from build123d import *

# Parameters (mm, degrees)
CUT_EXTRUDE2_DEPTH      = 87.677563418
CUT_EXTRUDE2_DEPTH_BACK = 87.677563418
SKETCH3_W               = 4
SKETCH3_H               = 2.8


with BuildPart() as part:
    # Sketch1 → Revolve1 (revolve)
    with BuildSketch(Plane.XY, mode=Mode.PRIVATE) as revolve1_sk:
        with BuildLine():
            Line((0, 0), (55, 0))
            Line((55, 0), (55, 8.5))
            Line((55, 8.5), (1, 8.5))
            ThreePointArc((1, 8.5), (0.292893219, 8.792893219), (0, 9.5))
            Line((0, 9.5), (0, 12))
            Line((0, 12), (-30, 12))
            Line((-30, 12), (-30, 9.5))
            ThreePointArc((-30, 9.5), (-30.292893219, 8.792893219), (-31, 8.5))
            Line((-31, 8.5), (-85, 8.5))
            Line((-85, 8.5), (-85, 0))
            Line((-85, 0), (0, 0))
        make_face()
    revolve(revolve1_sk.sketch.rotate(Axis((-85, 0, 0), (1, 0, 0)), 180), axis=Axis((-85, 0, 0), (1, 0, 0)))

    # Sketch3 → Cut-Extrude2 (cut, two sides: drawn at the far end of the back side and taken through both)
    with BuildSketch(Plane(origin=(0, 0, 0), x_dir=(0, 0, -1), z_dir=(1, 0, 0)).offset(-CUT_EXTRUDE2_DEPTH_BACK)):
        with Locations((2, 9.913708499)):
            Rectangle(SKETCH3_W, SKETCH3_H)
        with Locations((-2, 9.913708499)):
            Rectangle(SKETCH3_W, SKETCH3_H)
        with BuildLine():
            Line((-4, 11.313708499), (0, 11.313708499))
            Line((0, 11.313708499), (0, 12))
            ThreePointArc((0, 12), (-2.029223745, 11.827182716), (-4, 11.313708499))
        make_face()
        with BuildLine():
            Line((0, 12), (0, 11.313708499))
            Line((0, 11.313708499), (4, 11.313708499))
            ThreePointArc((4, 11.313708499), (2.029223745, 11.827182716), (0, 12))
        make_face()
    extrude(amount=CUT_EXTRUDE2_DEPTH + CUT_EXTRUDE2_DEPTH_BACK, mode=Mode.SUBTRACT)


solid = part.part
The listing builds one solid part. Answer for the finished solid, in the listing's coordinates (mm). A direction names the side the tool comes from. Round coordinates to 2 decimals unless told otherwise and drop trailing zeros. Order: outer loops, then holes, each group sorted by start corner. A loop starts at its lowest first (then second) coordinate and runs counter-clockwise, first axis right, second up. Notation, with made-up numbers: (17.5, -32.5) - (32.5, -32.5) arc R30 ccw to (32.5, -5.5) - close; hole circle Ø3 at (0, -7). An arc over 180 degrees is marked (long way). Write item = value, one per line. Start each with the question number.
1) Section C-C, the plane x = 25.5 is taken. Write down the section's boundary in (y, z), plus the area to 3 significant figures.
2) Section A-A, the plane y = 0 is taken. Write down the section's boundary in (x, z).
3) Given pin 1 (6 mm diameter, centred on x = 23, y = 4, fed in from +Z); pin 2 (1 mm diameter, centred on x = -60, z = 0, fed in from -Y); pin 3 (2.5 mm diameter, centred on x = -16.5, z = 1.5, fed in from +Y), each flat-ended and moving along its own axis, determine where each tip first touches the part or whether it passes through.
4) Section B-B, the plane z = 0 is taken. Write down the section's boundary in (x, y).
5) Straight lines are drawn through the part: L1, parallel to X at y = -9.75, z = -1.5; L2, parallel to Y at x = -57.5, z = -0.25; L3, parallel to Z at x = -27.5, y = 9.75. For each, find the intervals that lie inside material, in ascending order.
6) Section D-D, the plane x = -21.5 is taken. Write down the section's boundary in (y, z), plus the area to 3 significant figures.
7) For faces 4 (the flat face through (-15, 10, 4)), 5 (the cylindrical face through (27.622, 1.107, -8.428)), 6 (the cylindrical face through (-15, -12, 0)), 7 (the flat face through (-30, -9, -4)), 8 (the flat face through (55, 0, 0)), determine the directions among +Z, -Z, +X, -X, +Y, -Y from which every point of the face is accessible in a straight line to the end or side of a thin tool.
8) For a pull along Z with two mould halves and no side action, classify faces 1 (the flat face through (0, -9, 3.5)), 2 (the cylindrical face through (-58.378, 1.107, -8.428)), 3 (the flat face through (-15, 10, -4)) as released by +Z, released by -Z, zero draft, split by the parting line, or undercut.
Results list:
q1.outline = circle Ø17 at (0, 0)
q1.area = 227 mm^2
q2.outline = (-85, -8.5) - (-31, -8.5) arc R1 cw to (-30, -9.5) - (-30, -12) - (0, -12) - (0, -9.5) arc R1 cw to (1, -8.5) - (55, -8.5) - (55, 8.5) - (1, 8.5) arc R1 cw to (0, 9.5) - (0, 12) - (-30, 12) - (-30, 9.5) arc R1 cw to (-31, 8.5) - (-85, 8.5) - close
q3.pin_1 = 8.44
q3.pin_2 = -8.5
q3.pin_3 = 8.51
q4.outline = (-85, -8.5) - (-31, -8.5) arc R1 cw to (-30, -9.5) - (-30, -12) - (0, -12) - (0, -9.5) arc R1 cw to (1, -8.5) - (55, -8.5) - (55, 8.5) - (1, 8.5) arc R1 cw to (0.83, 8.51) - (-30.83, 8.51) arc R1 cw to (-31, 8.5) - (-85, 8.5) - close
q5.L1 = -30 to 0
q5.L2 = -8.5 to 8.5
q5.L3 = -7 to -4, 4 to 7
q6.outline = (8.51, -4) - (8.51, 4) - (11.31, 4) arc R12 ccw (long way) to (11.31, -4) - close
q6.area = 426 mm^2
q7.face_4 = +X, -X, +Y
q7.face_5 = +X
q7.face_6 = +X, -X
q7.face_7 = -X
q7.face_8 = +Z, -Z, +X, +Y, -Y
q8.face_1 = zero draft
q8.face_2 = split by the parting line
q8.face_3 = undercut
